Design review of the part built by this model. Coordinates are the model's own, in mm. Face numbers are marked on the shaded views. Round coordinates to 2 decimals unless told otherwise and drop trailing zeros. Write each loop counter-clockwise with the first axis right and the second up, starting at its lowest first coordinate (ties: lowest second). Pieces come first, ordered by that corner, then holes. Notation, with made-up numbers: (68.25, 13.25) -> (115.25, 13.25) arc R13 ccw to (115.25, 19.25) -> close; hole circle Ø11 at (36, -4). An arc over 180 degrees is marked (long way). One line per question, with ' | ' between items. Start each with the question number.
1) Insertion check: pin 1 Ø7 at (x, z) = (0, -55) entering from -Y; pin 2 Ø1 at (x, y) = (-20, -1.5) entering from +Z; pin 3 Ø12 at (y, z) = (-16.5, 6.5) entering from +X; pin 4 Ø4 at (x, y) = (-50, 17) entering from -Z. Each pin has a flat end and moves straight along its axis. Give the tip position at first contact, or say it passes through.
2) Consider section B-B (y = -0.5). Give the boundary of the cut face in (x, z).
3) Mouldability with a two-part tool opening along Z and no side actions: class the marked faces 1, 2 and 3 as +Z half, -Z half, draft (parallel to the pull), parting line (faces both ways), or undercut.
4) Consider section A-A (x = 0). Give the boundary of the cut face in (y, z).
5) For probe 1 along Y at (x, z) = (-46, 17); probe 2 along Z at (x, y) = (-55, 15); probe 3 along Z at (x, y) = (14.5, 8.5), list the stretches that pass through material, from the lowest coordinate up.
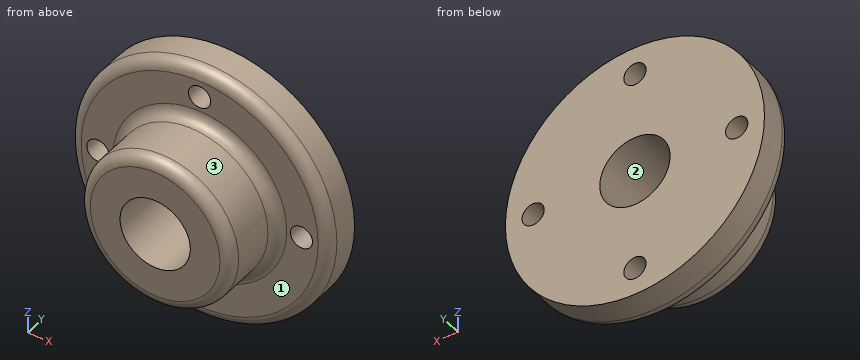
```python
from build123d import *

# Parameters (mm, degrees)
SKETCH2_R          = 6
CUT_EXTRUDE1_DEPTH = 106.000000067


with BuildPart() as part:
    # Sketch1 → Revolve1 (revolve)
    with BuildSketch(Plane.XY):
        with BuildLine():
            Line((70, 27.5), (19, 27.5))
            Line((19, 27.5), (19, -27.5))
            Line((19, -27.5), (35, -27.5))
            ThreePointArc((35, -27.5), (39.242640687, -25.742640687), (41, -21.5))
            Line((41, -21.5), (41, 1.5))
            ThreePointArc((41, 1.5), (42.757359313, 5.742640687), (47, 7.5))
            Line((47, 7.5), (64, 7.5))
            ThreePointArc((64, 7.5), (68.242640687, 9.257359313), (70, 13.5))
            Line((70, 13.5), (70, 27.5))
        make_face()
    revolve(axis=Axis((0, -27.5, 0), (0, 1, 0)))

    # Sketch2 → Cut-Extrude1 (cut, through all)
    with BuildSketch(Plane.XZ.offset(-7.5)):
        with Locations((-55, 0)):
            Circle(SKETCH2_R)
        with Locations((0, 55)):
            Circle(SKETCH2_R)
        with Locations((55, 0)):
            Circle(SKETCH2_R)
        with Locations((0, -55)):
            Circle(SKETCH2_R)
    extrude(amount=-CUT_EXTRUDE1_DEPTH, mode=Mode.SUBTRACT)


solid = part.part
```
From the geometry:
1) pin 1: passes through | pin 2: stops at z = 36.07 | pin 3: stops at x = 41 | pin 4: stops at z = -50.95
2) outline: circle Ø82 at (0, 0); hole circle Ø38 at (0, 0)
3) face 1: draft | face 2: undercut | face 3: parting line
4) outline: (-27.5, -35) arc R6 ccw to (-21.5, -41) -> (1.5, -41) arc R6 cw to (7.5, -47) -> (7.5, -49) -> (27.5, -49) -> (27.5, -19) -> (-27.5, -19) -> close; (-27.5, 19) -> (27.5, 19) -> (27.5, 49) -> (7.5, 49) -> (7.5, 47) arc R6 cw to (1.5, 41) -> (-21.5, 41) arc R6 ccw to (-27.5, 35) -> close; (7.5, -64) arc R6 ccw to (13.5, -70) -> (27.5, -70) -> (27.5, -61) -> (7.5, -61) -> close; (7.5, 61) -> (27.5, 61) -> (27.5, 70) -> (13.5, 70) arc R6 ccw to (7.5, 64) -> close
5) probe 1: y = 7.5 to 27.5 | probe 2: z = -43.3 to -6, 6 to 43.3 | probe 3: z = -65.74 to -12.28, 12.28 to 65.74
